The listing builds one solid part. Answer for the finished solid, in the listing's coordinates (mm). Face numbers are marked on the shaded views. A direction names the side the tool comes from. Give positions to 0.01 mm unless a question says otherwise; leave off trailing zeros. Write each loop counter-clockwise with the first axis right and the second up, starting at its lowest first coordinate (ties: lowest second). Pieces come first, ordered by that corner, then holes. Notation, with made-up numbers: (8.5, -16) - (15.5, -16) arc R24 ccw to (15.5, 23) - close; hole circle Ø8 at (81, -3.5). An arc over 180 degrees is marked (long way). Return JSON: item names as keys, results as strings.
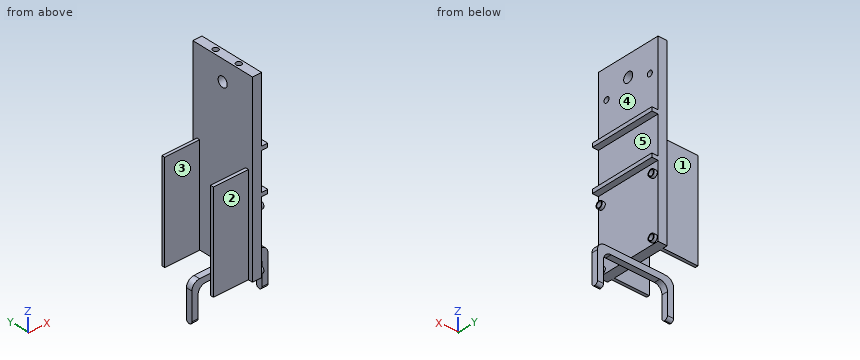
Autodesk Fusion 360 part; units mm, degrees
sketch "스케치1" plane through (0, 0, 0) normal (0, 1, 0) x (1, 0, 0)
  line L0 (-25, 0) -> (-25, -25)
  line L1 (-25, -25) -> (25, -25)
  line L2 (25, -25) -> (25, 0)
  line L3 (25, 0) -> (21, 0)
  line L4 (21, 0) -> (21, -21)
  line L5 (21, -21) -> (-21, -21)
  line L6 (-21, -21) -> (-21, 0)
  line L7 (-21, 0) -> (-25, 0)
extrude "돌출1" add sketch "스케치1" along normal mid plane 4
sketch "스케치2" plane through (0, 0, 25) normal (0, 0, 1) x (-1, 0, 0)
  line L0 (25, 2) -> (-25, 2)
  line L1 (3, -21.65) -> (-3, -21.65)
  line L2 (3, -21.65) -> (3, 0)
  line L3 (-3, -21.65) -> (-3, 0)
  line L4 (-20, 0) -> (-2.5, 0)
  line L5 (3, 21.65) -> (-3, 21.65)
  line L6 (3, 21.65) -> (3, 0)
  line L7 (-3, 21.65) -> (-3, 0)
  line L8 (25, -2) -> (-25, -2)
  dimension "d29" = 21.65
  dimension "d30" = 3
  dimension "d31" = 3
extrude "돌출2" add sketch "스케치2" along normal blind 120
sketch "스케치14" plane through (0, 0, 145) normal (0, 0, 1) x (-1, 0, 0)
  circle A0 centre (0, -8.4) radius 1.8
  line L0 (-1.75, 0) -> (-22.5, 0)
  circle A1 centre (0, 8.4) radius 1.8
  dimension "d34" = 3.6
  dimension "d35" = 8.4
extrude "돌출10" cut sketch "스케치14" against normal blind 4.7
thread "스레드1"
thread "스레드2"
sketch "스케치15" plane through (3, 0, 0) normal (1, 0, 0) x (0, 1, 0)
  line L0 (0, 1.75) -> (0, 22.5)
  line L1 (-21.65, 145) -> (21.65, 145)
  circle A0 centre (-18.85, 27.8) radius 2.25
  line L2 (2, 25) -> (21.65, 25)
  line L3 (-21.65, 25) -> (-21.65, 145)
  circle A1 centre (-18.85, 65.5) radius 2.25
  circle A2 centre (18.85, 65.5) radius 2.25
  circle A3 centre (18.85, 27.8) radius 2.25
  dimension "d43" = 4.5
  dimension "d44" = 2.8
  dimension "d45" = 2.8
  dimension "d46" = 4.5
  dimension "d47" = 37.7
extrude "돌출13" add sketch "스케치15" along normal blind 2
sketch "스케치17" plane through (5, 0, 0) normal (1, 0, 0) x (0, 1, 0)
  circle A0 centre (-18.85, 65.5) radius 1.8
  circle A1 centre (-18.85, 27.8) radius 1.8
  line L0 (0, 1.75) -> (0, 22.5)
  circle A2 centre (18.85, 27.8) radius 1.8
  circle A3 centre (18.85, 65.5) radius 1.8
  point P0 (-18.85, 65.5)
  point P1 (-18.85, 27.8)
  dimension "d56" = 3.6
  dimension "d57" = 3.6
extrude "돌출15" cut sketch "스케치17" against normal blind 4.7
thread "스레드7"
thread "스레드8"
thread "스레드9"
thread "스레드10"
sketch "스케치18" plane through (3, 0, 0) normal (1, 0, 0) x (0, 1, 0)
  line L0 (-21.65, 72.3985) -> (21.65, 72.3985)
  line L1 (21.65, 72.3985) -> (21.65, 74.8985)
  line L2 (21.65, 74.8985) -> (-21.65, 74.8985)
  line L3 (-21.65, 74.8985) -> (-21.65, 72.3985)
  line L4 (-21.65, 25) -> (-21.65, 145)
  line L5 (21.65, 25) -> (21.65, 145)
  line L6 (-21.65, 99.3985) -> (21.65, 99.3985)
  line L7 (21.65, 99.3985) -> (21.65, 101.8985)
  line L8 (21.65, 101.8985) -> (-21.65, 101.8985)
  line L9 (-21.65, 101.8985) -> (-21.65, 99.3985)
  dimension "d60" = 2.5
  dimension "d61" = 2.5
  dimension "d62" = 24.5
extrude "돌출16" add sketch "스케치18" along normal blind 4 contours L0 L1 L2 L3 L4 L5 | L4 L5 L6 L7 L8 L9
sketch "스케치19" plane through (3, 0, 0) normal (1, 0, 0) x (0, 1, 0)
  circle A0 centre (0, 126) radius 12
  circle A1 centre (15.7, 126) radius 1.8
  line L0 (0, 2.5) -> (0, 20)
  circle A2 centre (-15.7, 126) radius 1.8
  circle A3 centre (0, 131.5) radius 3.3
  circle A4 centre (0, 131.5) radius 1.8
  dimension "d65" = 24
  dimension "d66" = 3.6
  dimension "d67" = 15.7
  dimension "d68" = 6.6
  dimension "d69" = 5.5
  dimension "d70" = 3.6
extrude "돌출17" cut sketch "스케치19" against normal blind 4.7 contours A1 | A2
extrude "돌출18" cut sketch "스케치19" against normal through all contours A3 | A4
sketch "스케치20" plane through (-3, 0, 0) normal (-1, 0, 0) x (0, -1, 0)
  line L0 (-2, 25) -> (-21.65, 25)
  line L1 (-16.65, 25) -> (-16.65, 89.5)
  line L2 (16.65, 25) -> (16.65, 89.5)
  line L3 (-16.65, 89.5) -> (-18.65, 89.5)
  line L4 (-18.65, 89.5) -> (-18.65, 25)
  line L5 (-18.65, 25) -> (-16.65, 25)
  line L6 (16.65, 25) -> (18.65, 25)
  line L7 (18.65, 25) -> (18.65, 89.5)
  line L8 (18.65, 89.5) -> (16.65, 89.5)
  point P0 (21.65, 25)
  dimension "d74" = 33.3
  dimension "d75" = 5
  dimension "d76" = 5
  dimension "d77" = 2
  dimension "d78" = 2
  dimension "d79" = 64.5
extrude "돌출19" add sketch "스케치20" along normal blind 23
fillet "모깎기1" radius 5 4 edges at (-21, 0, 21) (-25, 0, 25) (21, 0, 21) (25, 0, 25)
fillet "모깎기2" radius 2 4 edges at (-23, -2, 0) (-23, 2, 0) (23, -2, 0) (23, 2, 0)
equation "d35 = 10 mm - 1.6 mm"
equation "d67 = 18.5 mm - 2.8 mm"
equation "d69 = 8.5 mm - 3 mm"
Item 1: For the marked faces 1, 2 and 3, determine the directions among +Z, -Z, +X, -X, +Y, -Y from which every point of the face is accessible in a straight line to the end or side of a thin tool.
Answer below:
{"face 1": "+Z, -Z, -X, +Y", "face 2": "+Z, -Z, -X, -Y", "face 3": "+Z, -Z, -X"}
Item 2: A cutting plane is placed at A-A on x = -11.5. Determine the outline of the cut face in (y, z).
Answer below:
{"outline": "(-18.65, 25) - (-16.65, 25) - (-16.65, 89.5) - (-18.65, 89.5) - close; (-2, 21) - (2, 21) - (2, 25) - (-2, 25) - close; (16.65, 25) - (18.65, 25) - (18.65, 89.5) - (16.65, 89.5) - close"}
Item 3: A cutting plane is placed at B-B on z = 131.5. Determine the outline of the cut face in (x, y).
Answer below:
{"outline": "(-3, -21.65) - (3, -21.65) - (3, -3.3) - (-3, -3.3) - close; (-3, 3.3) - (3, 3.3) - (3, 21.65) - (-3, 21.65) - close"}
Item 4: Flat-ended cylindrical pins translate along their axes: P1, Ø18.5, axis at x = -12, z = 8, coming from the -Y side; P2, Ø1.1, axis at y = 19, z = 28, coming from the +X side; P3, Ø21.5, axis at y = -3.5, z = 128.5, coming from the +X side; P4, Ø6, axis at y = 18.85, z = 65.5, coming from the -X side. Find the tip coordinate at first contact, or state that the pin passes through.
Answer below:
{"P1": "stops at y = -2", "P2": "stops at x = 0.3", "P3": "stops at x = 3", "P4": "stops at x = -26"}
Item 5: The mould has two halves that part along Z. Classify the marked faces 4 and 5: +Z half, -Z half, draft (parallel to the pull), parting line (faces both ways), or undercut.
Answer below:
{"face 4": "draft", "face 5": "undercut"}
Item 6: Consider L1, parallel to Y at x = 0.85, z = 126; L2, parallel to X at y = -8.4, z = 142.5; L3, parallel to Y at x = -4.5, z = 64. Determine where each line is inside the solid, lowest interval first.
Answer below:
{"L1": "y = -21.65 to -17.5, -13.9 to 13.9, 17.5 to 21.65", "L2": "x = -3 to -1.8, 1.8 to 3", "L3": "y = -18.65 to -16.65, 16.65 to 18.65"}
Item 7: A cutting plane is placed at C-C on z = 53. Determine the outline of the cut face in (x, y).
Answer below:
{"outline": "(-26, -18.65) - (-3, -18.65) - (-3, -21.65) - (3, -21.65) - (3, 21.65) - (-3, 21.65) - (-3, 18.65) - (-26, 18.65) - (-26, 16.65) - (-3, 16.65) - (-3, -16.65) - (-26, -16.65) - close"}
Item 8: A cutting plane is placed at D-D on y = -8.4. Determine the outline of the cut face in (x, z), then the cut area to 3 significant figures.
Answer below:
{"outline": "(-3, 25) - (3, 25) - (3, 72.4) - (7, 72.4) - (7, 74.9) - (3, 74.9) - (3, 99.4) - (7, 99.4) - (7, 101.9) - (3, 101.9) - (3, 145) - (1.8, 145) - (1.8, 140.3) - (-1.8, 140.3) - (-1.8, 145) - (-3, 145) - close", "area": "723 mm²"}
